Input: part model. Units: mm. Frame: model coordinates. Coordinates: 2 decimals unless noted, no trailing zeros. Loops run counter-clockwise (first coordinate to the right, second up) from the corner with the lowest first, then second, coordinate; pieces in that order, holes last.
```python
from build123d import *

# Parameters (mm, degrees)
SKETCH1_R           = 177
BOSS_EXTRUDE1_DEPTH = 4.7625
SKETCH2_R           = 1.7
CUT_EXTRUDE1_DEPTH  = 251.361102023
SKETCH3_R           = 2.667
ZIP_TIES_DEPTH      = 251.361102023
SKETCH4_R           = 10.16
WIRES_2_DEPTH       = 251.361102023


with BuildPart() as part:
    # Sketch1 → Boss-Extrude1 (new body)
    with BuildSketch(Plane(origin=(0, 0, 0), x_dir=(1, 0, 0), z_dir=(0, 1, 0))):
        with Locations(Location((0, 0, 0), (0, 0, 90))):
            Circle(SKETCH1_R)
    extrude(amount=BOSS_EXTRUDE1_DEPTH)

    # Sketch2 → Cut-Extrude1 (cut, through all)
    with BuildSketch(Plane(origin=(0, 4.7625, 0), x_dir=(1, 0, 0), z_dir=(0, 1, 0))):
        with Locations(Location((142.287973842, -82.15, 0), (0, 0, 270))):
            Circle(SKETCH2_R)
        with Locations(Location((134.039081871, -86.9125, 0), (0, 0, 270))):
            Circle(SKETCH2_R)
        with Locations(Location((125.7901899, -82.15, 0), (0, 0, 270))):
            Circle(SKETCH2_R)
        with Locations(Location((125.7901899, -72.625, 0), (0, 0, 270))):
            Circle(SKETCH2_R)
        with Locations(Location((134.039081871, -67.8625, 0), (0, 0, 270))):
            Circle(SKETCH2_R)
        with Locations(Location((142.287973842, -72.625, 0), (0, 0, 270))):
            Circle(SKETCH2_R)
        with Locations(Location((-142.287973842, -72.625, 0), (0, 0, 270))):
            Circle(SKETCH2_R)
        with Locations(Location((-134.039081871, -67.8625, 0), (0, 0, 270))):
            Circle(SKETCH2_R)
        with Locations(Location((-125.7901899, -72.625, 0), (0, 0, 270))):
            Circle(SKETCH2_R)
        with Locations(Location((-125.7901899, -82.15, 0), (0, 0, 270))):
            Circle(SKETCH2_R)
        with Locations(Location((-134.039081871, -86.9125, 0), (0, 0, 270))):
            Circle(SKETCH2_R)
        with Locations(Location((-142.287973842, -82.15, 0), (0, 0, 270))):
            Circle(SKETCH2_R)
        with Locations(Location((-142.287973842, 82.15, 0), (0, 0, 270))):
            Circle(SKETCH2_R)
        with Locations(Location((-134.039081871, 86.9125, 0), (0, 0, 270))):
            Circle(SKETCH2_R)
        with Locations(Location((-125.7901899, 82.15, 0), (0, 0, 270))):
            Circle(SKETCH2_R)
        with Locations(Location((-125.7901899, 72.625, 0), (0, 0, 270))):
            Circle(SKETCH2_R)
        with Locations(Location((-134.039081871, 67.8625, 0), (0, 0, 270))):
            Circle(SKETCH2_R)
        with Locations(Location((-142.287973842, 72.625, 0), (0, 0, 270))):
            Circle(SKETCH2_R)
        with Locations(Location((142.287973842, 72.625, 0), (0, 0, 270))):
            Circle(SKETCH2_R)
        with Locations(Location((134.039081871, 67.8625, 0), (0, 0, 270))):
            Circle(SKETCH2_R)
        with Locations(Location((125.7901899, 72.625, 0), (0, 0, 270))):
            Circle(SKETCH2_R)
        with Locations(Location((125.7901899, 82.15, 0), (0, 0, 270))):
            Circle(SKETCH2_R)
        with Locations(Location((134.039081871, 86.9125, 0), (0, 0, 270))):
            Circle(SKETCH2_R)
        with Locations(Location((142.287973842, 82.15, 0), (0, 0, 270))):
            Circle(SKETCH2_R)
    extrude(amount=-CUT_EXTRUDE1_DEPTH, mode=Mode.SUBTRACT)

    # Sketch3 → Zip Ties (cut, through all)
    with BuildSketch(Plane(origin=(0, 4.7625, 0), x_dir=(1, 0, 0), z_dir=(0, 1, 0))):
        with Locations(Location((0, -141.44, 0), (0, 0, 270))):
            Circle(SKETCH3_R)
        with Locations(Location((-100.013183131, -100.013183131, 0), (0, 0, 270))):
            Circle(SKETCH3_R)
        with Locations(Location((-141.44, 0, 0), (0, 0, 270))):
            Circle(SKETCH3_R)
        with Locations(Location((-100.013183131, 100.013183131, 0), (0, 0, 270))):
            Circle(SKETCH3_R)
        with Locations(Location((0, 141.44, 0), (0, 0, 270))):
            Circle(SKETCH3_R)
        with Locations(Location((100.013183131, 100.013183131, 0), (0, 0, 270))):
            Circle(SKETCH3_R)
        with Locations(Location((141.44, 0, 0), (0, 0, 270))):
            Circle(SKETCH3_R)
        with Locations(Location((100.013183131, -100.013183131, 0), (0, 0, 270))):
            Circle(SKETCH3_R)
    extrude(amount=-ZIP_TIES_DEPTH, mode=Mode.SUBTRACT)

    # Sketch4 → Wires 2 (cut, through all)
    with BuildSketch(Plane(origin=(0, 4.7625, 0), x_dir=(1, 0, 0), z_dir=(0, 1, 0))):
        with Locations(Location((-127, 50.8, 0), (0, 0, 270))):
            Circle(SKETCH4_R)
        with Locations(Location((127, 50.8, 0), (0, 0, 270))):
            Circle(SKETCH4_R)
    extrude(amount=-WIRES_2_DEPTH, mode=Mode.SUBTRACT)


solid = part.part
```
Item 1: Section query D-D (x = 108.5). Output: boundary loops of the cut face in (y, z).
Result:
outline: (0, -139.85) - (4.76, -139.85) - (4.76, 139.85) - (0, 139.85) - close
Item 2: Contact query for flat-ended pins moving along their axis: P1, Ø1, axis at x = -104, y = 0.5, coming from the +Z side; P2, Ø1.5, axis at y = 3.5, z = 110.5, coming from the -X side; P3, Ø2.5, axis at x = 142.29, z = 72.62, coming from the -Y side (3 decimals); P4, Ø2, axis at y = 4, z = -32.5, coming from the +X side. Output: stop coordinate, or through.
Result:
P1: stops at z = 143.59
P2: stops at x = -138.87
P3: passes through
P4: stops at x = 174.17
Item 3: Mould query, pull axis Z, two halves, no side actions, for faces 1 (the face through (-120.133, 2.415, -58.288)), 2 (the face through (172.79, 2.35, 38.37)), 3 (the face through (-2, 0, 2)). Classes: +Z half, -Z half, draft (parallel to the pull), parting line (faces both ways), or undercut.
Result:
face 1: undercut
face 2: parting line
face 3: draft
Item 4: Section query A-A (z = -50.8). Output: boundary loops of the cut face in (x, y).
Result:
outline: (-169.55, 0) - (-137.16, 0) - (-137.16, 4.76) - (-169.55, 4.76) - close; (-116.84, 0) - (116.84, 0) - (116.84, 4.76) - (-116.84, 4.76) - close; (137.16, 0) - (169.55, 0) - (169.55, 4.76) - (137.16, 4.76) - close
Item 5: Line query: L1, parallel to Z at x = -101, y = 0.7; L2, parallel to X at y = 0.9, z = -53; L3, parallel to Z at x = -141.44, y = 3.55. Output: solid intervals per line, ascending.
Result:
L1: z = -145.35 to -102.49, -97.54 to 97.54, 102.49 to 145.35
L2: x = -168.88 to -136.92, -117.08 to 117.08, 136.92 to 168.88
L3: z = -106.41 to -83.62, -80.68 to -74.1, -71.15 to -2.67, 2.67 to 71.15, 74.1 to 80.68, 83.62 to 106.41
Item 6: Section query C-C (x = 44). Output: boundary loops of the cut face in (y, z).
Result:
outline: (0, -171.44) - (4.76, -171.44) - (4.76, 171.44) - (0, 171.44) - close
Item 7: Section query B-B (y = 3.5). Count the separate pieces of the cut face and the enclosed holes in it, then the cut area to 3 significant figures.
Result:
separate pieces: 1
enclosed holes: 34
area: 97,400 mm2
